```python
from build123d import *

# Parameters (mm, degrees)
SKETCH_1_W             = 28
SKETCH_1_H             = 16
EXTRUDE_1_DEPTH        = 5
FILLET_1_R             = 3
CUT_EXTRUDE_2_DEPTH    = 0.8
FILLET_2_R             = 3
FILLET_2_OF_MIRROR_1_R = 3
SKETCH_3_R             = 1.5
CUT_EXTRUDE_3_DEPTH    = 19.973665961
SKETCH_4_R             = 2
CUT_EXTRUDE_4_DEPTH    = 0.5
CUT_EXTRUDE_START      = -1
SKETCH_5_R             = 2
CUT_EXTRUDE_5_DEPTH    = 1
SKETCH_10_W            = 6.5
SKETCH_10_H            = 0.5
EXTRUDE_9_DEPTH        = 10
SKETCH_11_W            = 6.5
SKETCH_11_H            = 1
CUT_EXTRUDE_10_DEPTH   = 27.669270706
CHAMFER_1_SIZE         = 1
EXTRUDE_11_DEPTH       = 3.25
FILLET_7_R             = 0.5
SKETCH_13_W            = 5.5
SKETCH_13_H            = 1
CUT_EXTRUDE_12_DEPTH   = 3
CHAMFER_2_SIZE         = 1
SKETCH_14_W            = 2.8
SKETCH_14_H            = 4
EXTRUDE_13_DEPTH       = 3
FILLET_8_R             = 1.4


with BuildPart() as part:
    # 草圖1 → 伸長1 (new, symmetric)
    with BuildSketch(Plane.XY):
        Rectangle(SKETCH_1_W, SKETCH_1_H)
    extrude(amount=EXTRUDE_1_DEPTH, both=True)

    # 圓角1
    fillet_1_edges = [part.edges().sort_by_distance(p)[0] for p in [
        (-14, 8, 0),
        (14, 8, 0),
        (14, -8, 0),
        (-14, -8, 0),
    ]]
    fillet(fillet_1_edges, radius=FILLET_1_R)

    # 草圖2 → 伸長2 (cut)
    with BuildSketch(Plane.XY.offset(5)):
        with BuildLine():
            Line((-14, -2.5), (-8.5, -2.5))
            Line((-8.5, -2.5), (-8.5, -8))
            Line((-8.5, -8), (11, -8))
            ThreePointArc((11, -8), (13.121320344, -7.121320344), (14, -5))
            Line((14, -5), (14, 2.5))
            Line((14, 2.5), (8.5, 2.5))
            Line((8.5, 2.5), (8.5, 8))
            Line((8.5, 8), (-11, 8))
            ThreePointArc((-11, 8), (-13.121320344, 7.121320344), (-14, 5))
            Line((-14, 5), (-14, -2.5))
        make_face()
    cut_extrude_2 = extrude(amount=-CUT_EXTRUDE_2_DEPTH, mode=Mode.SUBTRACT)

    # 圓角2
    fillet_2_edges = [part.edges().sort_by_distance(p)[0] for p in [
        (8.5, 2.5, 4.6),
        (-8.5, -2.5, 4.6),
    ]]
    fillet(fillet_2_edges, radius=FILLET_2_R)

    # 鏡射1: 伸長2 across plane
    add(cut_extrude_2.mirror(Plane.XY), mode=Mode.SUBTRACT)

    # 圓角2 of 鏡射1
    fillet_2_of_mirror_1_edges = [part.edges().sort_by_distance(p)[0] for p in [
        (8.5, 2.5, -4.6),
        (-8.5, -2.5, -4.6),
    ]]
    fillet(fillet_2_of_mirror_1_edges, radius=FILLET_2_OF_MIRROR_1_R)

    # 草圖3 → 伸長3 (cut, through all)
    with BuildSketch(Plane(origin=(0, 0, -5), x_dir=(-1, 0, 0), z_dir=(0, 0, -1))):
        with Locations((-11.5, 5)):
            Circle(SKETCH_3_R)
        with Locations((11.5, -5)):
            Circle(SKETCH_3_R)
    extrude(amount=-CUT_EXTRUDE_3_DEPTH, mode=Mode.SUBTRACT)

    # 草圖4 → 伸長4 (cut)
    with BuildSketch(Plane(origin=(0, 0, -4.2), x_dir=(-1, 0, 0), z_dir=(0, 0, -1))):
        with Locations((0, 5.5)):
            Circle(SKETCH_4_R)
    extrude(amount=-CUT_EXTRUDE_4_DEPTH, mode=Mode.SUBTRACT)

    # 草圖5 → 伸長5 (cut)
    with BuildSketch(Plane.XY.offset(4.2).offset(CUT_EXTRUDE_START)):
        with Locations(Location((0, 5.5, 0), (0, 0, 180))):
            Circle(SKETCH_5_R)
    extrude(amount=CUT_EXTRUDE_5_DEPTH, mode=Mode.SUBTRACT)

    # 草圖9 → 旋轉1 (revolve)
    with BuildSketch(Plane(origin=(0, 5.5, 0), x_dir=(-1, 0, 0), z_dir=(0, 1, 0)), mode=Mode.PRIVATE) as revolve_1_sk:
        with BuildLine():
            Line((0, 3.2), (2, 3.2))
            ThreePointArc((2, 3.2), (1.077032961, 3.792582404), (0, 4))
            Line((0, 4), (0, 3.2))
        make_face()
    revolve(revolve_1_sk.sketch.rotate(Axis((0, 5.5, 3.2), (0, 0, 1)), 180), axis=Axis((0, 5.5, 3.2), (0, 0, 1)))

    # 草圖10 → 伸長9 (add)
    with BuildSketch(Plane(origin=(14, 0, 0), x_dir=(0, 0, -1), z_dir=(1, 0, 0))):
        with Locations((0, -3.75)):
            Rectangle(SKETCH_10_W, SKETCH_10_H)
        with Locations((0, 2.25)):
            Rectangle(SKETCH_10_W, SKETCH_10_H)
    extrude(amount=EXTRUDE_9_DEPTH)

    # 草圖11 → 伸長10 (cut, through all)
    with BuildSketch(Plane(origin=(0, 2.5, 0), x_dir=(1, 0, 0), z_dir=(0, 1, 0))):
        with BuildLine():
            Line((20.068181818, 1.071272126), (21.022727273, 0.698655734))
            ThreePointArc((21.022727273, 0.698655734), (21.5, 0), (21.022727273, -0.698655734))
            Line((21.022727273, -0.698655734), (20.068181818, -1.071272126))
            ThreePointArc((20.068181818, -1.071272126), (18.5, 0), (20.068181818, 1.071272126))
        make_face()
        with Locations((20.75, 2.75)):
            Rectangle(SKETCH_11_W, SKETCH_11_H)
        with Locations((20.75, -2.75)):
            Rectangle(SKETCH_11_W, SKETCH_11_H)
    extrude(amount=-CUT_EXTRUDE_10_DEPTH, mode=Mode.SUBTRACT)

    # 導角1
    chamfer_1_edges = [part.edges().sort_by_distance(p)[0] for p in [
        (24, 2.25, -2.25),
        (24, -3.75, -2.25),
        (24, 2.25, 2.25),
        (24, -3.75, 2.25),
    ]]
    chamfer(chamfer_1_edges, length=CHAMFER_1_SIZE)

    # 草圖12 → 伸長11 (add, symmetric)
    with BuildSketch(Plane.XY):
        Polygon((1, -8), (1.5, -8), (1.5, -10.5), (10.3, -10.5), (10.3, -11), (1, -11), align=None)
    extrude(amount=EXTRUDE_11_DEPTH, both=True)

    # 圓角7
    fillet_7_edges = [part.edges().sort_by_distance(p)[0] for p in [
        (1, -11, 0),
    ]]
    fillet(fillet_7_edges, radius=FILLET_7_R)

    # 草圖13 → 伸長12 (cut)
    with BuildSketch(Plane.XZ.offset(11)):
        with Locations((7.55, 2.75)):
            Rectangle(SKETCH_13_W, SKETCH_13_H)
        with Locations((7.55, -2.75)):
            Rectangle(SKETCH_13_W, SKETCH_13_H)
        with BuildLine():
            Line((6.368181818, 1.071272126), (7.322727273, 0.698655734))
            ThreePointArc((7.322727273, 0.698655734), (7.8, 0), (7.322727273, -0.698655734))
            Line((7.322727273, -0.698655734), (6.368181818, -1.071272126))
            ThreePointArc((6.368181818, -1.071272126), (4.8, 0), (6.368181818, 1.071272126))
        make_face()
    extrude(amount=-CUT_EXTRUDE_12_DEPTH, mode=Mode.SUBTRACT)

    # 導角2
    chamfer_2_edges = [part.edges().sort_by_distance(p)[0] for p in [
        (10.3, -10.75, 2.25),
        (10.3, -10.75, -2.25),
    ]]
    chamfer(chamfer_2_edges, length=CHAMFER_2_SIZE)

    # 草圖14 → 伸長13 (add)
    with BuildSketch(Plane(origin=(0, 8, 0), x_dir=(1, 0, 0), z_dir=(0, 1, 0))):
        with Locations((-9.6, 0)):
            Rectangle(SKETCH_14_W, SKETCH_14_H)
    extrude(amount=EXTRUDE_13_DEPTH)

    # 圓角8
    fillet_8_edges = [part.edges().sort_by_distance(p)[0] for p in [
        (-8.2, 11, 0),
        (-11, 11, 0),
    ]]
    fillet(fillet_8_edges, radius=FILLET_8_R - 0.0001)  # a hair under: the kernel refuses the full size


solid = part.part
```
The listing builds one solid part. Answer for the finished solid, in the listing's coordinates (mm). A direction names the side the tool comes from. Coordinates: 2 decimals unless noted, no trailing zeros. Write each loop counter-clockwise with the first axis right and the second up, starting at its lowest first coordinate (ties: lowest second). Pieces come first, ordered by that corner, then holes. Notation, with made-up numbers: M 76,89 L 128,89 A36 ccw 128,123 Z; hole C -16.5,50 d10. An arc over 180 degrees is marked long. Use a Markdown table: item, result. Add a question column.
1. Section C-C (x = 12) is taken. Give the vertices of the cut face in (y, z), plus the area to 3 significant figures.
2. Which of the six approach directions +Z, -Z, +X, -X, +Y, -Y give full straight-line access (tool end or side, diameter ignored) to faces 1 (the flat face through (-11, 9, 0)), 2 (the flat face through (9.81, -10.75, 1.74)), 3 (the flat face through (-10, 9, 2)), 4 (the flat face through (18, -3.5, 0)), 5 (the flat face through (-10, 9, -2))?
3. Given P1, Ø3, axis at x = 5.5, z = 0.5, coming from the -Y side; P2, Ø2, axis at x = 17, z = 1.5, coming from the -Y side; P3, Ø1, axis at x = -10, y = -1, coming from the -Z side; P4, Ø2, axis at x = 11.5, z = -2, coming from the -Y side, each flat-ended and moving along its own axis, determine where each tip first touches the part or whether it passes through.
4. Straight lines are drawn through the part: line 1 along X through (y, z) = (2.15, 0); line 2 along Z through (x, y) = (8.5, -7.5); line 3 along X through (y, z) = (6.25, -4.25). For each, find the intervals that lie inside material, in ascending order. Write a range as [from, to].
5. Section A-A (x = 19.65) is taken. Give the vertices of the cut face in (y, z).
6. Section D-D (x = 0) is taken. Give the vertices of the cut face in (y, z).
7. For a pull along X with two mould halves and no side action, classify faces 6 (the flat face through (2.5, -10.7, 3.25)), 7 (the cylindrical face through (0.26, 7.483, -3.954)), 8 (the flat face through (1.5, -9, 0)) as +X half, -X half, draft (parallel to the pull), parting line (faces both ways), or undercut.
8. Section B-B (z = 0) is taken. Count the separate pieces of the cut face and the enclosed holes in it, plus the area to 3 significant figures.
Data:
| question | item | result |
|---|---|---|
| 1 | outline | M -7.83,-4.2 L 2.5,-4.2 L 2.5,-5 L 3.59,-5 L 3.59,5 L 2.5,5 L 2.5,4.2 L -7.83,4.2 Z; M 6.41,-5 L 7.83,-5 L 7.83,5 L 6.41,5 Z |
| 1 | area | 112 mm2 |
| 2 | face 1 | +Z, -Z, -X, +Y |
| 2 | face 2 | +Z, +X, -Y |
| 2 | face 3 | +Z, +X, -X, +Y |
| 2 | face 4 | +Z, -Z, +X |
| 2 | face 5 | -Z, +X, -X, +Y |
| 3 | P1 | stops at y = -11 |
| 3 | P2 | stops at y = -4 |
| 3 | P3 | stops at z = -4.2 |
| 3 | P4 | stops at y = -8 |
| 4 | line 1 | x = [-14, 18.5], [21.5, 24] |
| 4 | line 2 | z = [-4.2, 4.2] |
| 4 | line 3 | x = [8.5, 10.67], [12.33, 13.73] |
| 5 | outline | M -4,-2.25 L -3.5,-2.25 L -3.5,-1.15 L -4,-1.15 Z; M -4,1.15 L -3.5,1.15 L -3.5,2.25 L -4,2.25 Z; M 2,-2.25 L 2.5,-2.25 L 2.5,-1.15 L 2,-1.15 Z; M 2,1.15 L 2.5,1.15 L 2.5,2.25 L 2,2.25 Z |
| 6 | outline | M -8,-4.2 L 3.5,-4.2 L 3.5,-3.7 L 7.5,-3.7 L 7.5,-4.2 L 8,-4.2 L 8,4.2 L 7.5,4.2 L 7.5,3.2 A2.9 ccw 3.5,3.2 L 3.5,4.2 L -8,4.2 Z |
| 7 | face 6 | draft |
| 7 | face 7 | undercut |
| 7 | face 8 | +X half |
| 8 | separate pieces | 4 |
| 8 | enclosed holes | 2 |
| 8 | area | 445 mm2 |
